from build123d import *

# Parameters (mm, degrees)
F1_DEPTH = 400


with BuildPart() as f1:
    # F0 (on Front) → F1 (new body)
    with BuildSketch(Plane.XZ):
        with BuildLine():
            Line((-35.55349, -68.947688), (-97.55349, -68.947688))
            Line((-97.55349, -68.947688), (-97.55349, -77.947688))
            Line((-97.55349, -77.947688), (62.44651, -77.947688))
            Line((62.44651, -77.947688), (62.44651, -68.947688))
            Line((62.44651, -68.947688), (0.44651, -68.947688))
            ThreePointArc((0.44651, -68.947688), (-10.160092, -64.55429), (-14.55349, -53.947688))
            Line((-14.55349, -53.947688), (-14.55349, 50.052312))
            ThreePointArc((-14.55349, 50.052312), (-10.160092, 60.658913), (0.44651, 65.052312))
            Line((0.44651, 65.052312), (62.44651, 65.052312))
            Line((62.44651, 65.052312), (62.44651, 74.052312))
            Line((62.44651, 74.052312), (-97.55349, 74.052312))
            Line((-97.55349, 74.052312), (-97.55349, 65.052312))
            Line((-97.55349, 65.052312), (-35.55349, 65.052312))
            ThreePointArc((-35.55349, 65.052312), (-24.946889, 60.658913), (-20.55349, 50.052312))
            Line((-20.55349, 50.052312), (-20.55349, -53.947688))
            ThreePointArc((-20.55349, -53.947688), (-24.946889, -64.55429), (-35.55349, -68.947688))
        make_face()
    extrude(amount=F1_DEPTH)


solid = f1.part
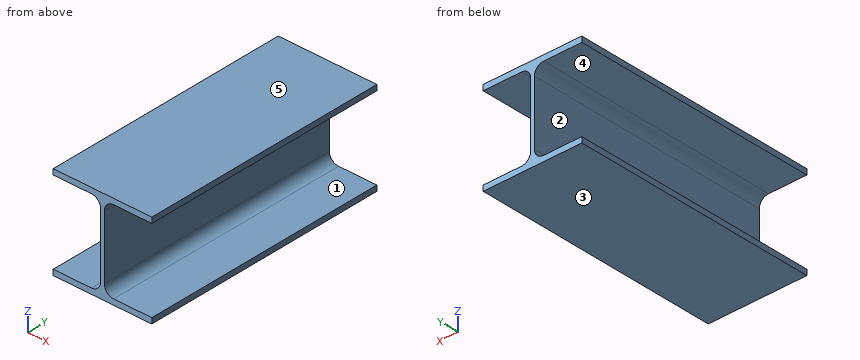
The listing builds one solid part. Answer for the finished solid, in the listing's coordinates (mm). Face numbers are marked on the shaded views. A direction names the side the tool comes from. Give positions to 0.01 mm unless a question says otherwise; leave off trailing zeros. Write each loop counter-clockwise with the first axis right and the second up, starting at its lowest first coordinate (ties: lowest second). Pieces come first, ordered by that corner, then holes. Notation, with made-up numbers: (78.25, 27.5) - (108.25, 27.5) arc R12 cw to (108.25, 33.5) - close; hole circle Ø10 at (64, 60). An arc over 180 degrees is marked (long way). Use a Markdown table: item, result.
1. Section B-B on y = -212.5 is taken. Write down the section's boundary in (x, z), plus the area to 3 significant figures.
Values follow:
| item | result |
|---|---|
| outline | (-97.55, -77.95) - (62.45, -77.95) - (62.45, -68.95) - (0.45, -68.95) arc R15 cw to (-14.55, -53.95) - (-14.55, 50.05) arc R15 cw to (0.45, 65.05) - (62.45, 65.05) - (62.45, 74.05) - (-97.55, 74.05) - (-97.55, 65.05) - (-35.55, 65.05) arc R15 cw to (-20.55, 50.05) - (-20.55, -53.95) arc R15 cw to (-35.55, -68.95) - (-97.55, -68.95) - close |
| area | 3,880 mm² |
2. For a pull along Z with two mould halves and no side action, classify the marked faces 3, 4 and 5 as released by +Z, released by -Z, zero draft, split by the parting line, or undercut.
Values follow:
| item | result |
|---|---|
| face 3 | released by -Z |
| face 4 | undercut |
| face 5 | released by +Z |
3. Each of these flat-tipped pins is pushed along its axis until it touches: P1, Ø2, axis at x = -21, z = -36, coming from the +Y side; P2, Ø5, axis at y = -357, z = -57, coming from the -X side; P3, Ø8, axis at y = -142, z = -2.5, coming from the +X side. Where does it stop, or does it pass through?
Values follow:
| item | result |
|---|---|
| P1 | stops at y = 0 |
| P2 | stops at x = -21.62 |
| P3 | stops at x = -14.55 |
4. A tool of negligible diameter and unlimited length cuts with its end or side. For the marked faces 1 and 2, from which of +Z, -Z, +X, -X, +Y, -Y can it reach the whole face along a straight path? Write none if from no direction.
Values follow:
| item | result |
|---|---|
| face 1 | +X, +Y, -Y |
| face 2 | -X, +Y, -Y |
5. Section C-C on z = -43 is taken. Write down the section's boundary in (x, y), plus the area to 3 significant figures.
Values follow:
| item | result |
|---|---|
| outline | (-20.55, -400) - (-14.55, -400) - (-14.55, 0) - (-20.55, 0) - close |
| area | 2,400 mm² |
6. Section A-A on x = -56.5 is taken. Write down the section's boundary in (y, z), plus the area to 3 significant figures.
Values follow:
| item | result |
|---|---|
| outline | (-400, -77.95) - (0, -77.95) - (0, -68.95) - (-400, -68.95) - close; (-400, 65.05) - (0, 65.05) - (0, 74.05) - (-400, 74.05) - close |
| area | 7,200 mm² |
7. Find the intervals of material crossed by probe 1 along Z at (x, y) = (51.5, -88); probe 2 along X at (y, z) = (-337.5, -54); probe 3 along X at (y, z) = (-271.5, -56), in increasing order. Write a range as from..to.
Values follow:
| item | result |
|---|---|
| probe 1 | z = -77.95..-68.95, 65.05..74.05 |
| probe 2 | x = -20.55..-14.55 |
| probe 3 | x = -20.69..-14.41 |
8. Section D-D on x = -28 is taken. Write down the section's boundary in (y, z), plus the area to 3 significant figures.
Values follow:
| item | result |
|---|---|
| outline | (-400, -77.95) - (0, -77.95) - (0, -66.91) - (-400, -66.91) - close; (-400, 63.01) - (0, 63.01) - (0, 74.05) - (-400, 74.05) - close |
| area | 8,830 mm² |
